from build123d import *

# Parameters (mm, degrees)
F1_DEPTH  = 20
F3_DEPTH  = 4
F5_DEPTH  = 1
F7_DEPTH  = 20.001
F10_W     = 15
F10_H     = 9.1
F11_DEPTH = 1
F8_R      = 3.75
F12_DEPTH = 10


# Not quite as in the source:
# - a pattern or mirror of a feature is missing from the dataset's text; its kind, count and spacing are read off the source's solid


with BuildPart() as f1:
    # F0 (on Front) → F1 (new body)
    with BuildSketch(Plane.XZ):
        Polygon((-16.45, 3), (-19.25, -1.7), (-18.09, -1.7), (-17.0772340426, 0), (0, 0), (0, 3), align=None)
    extrude(amount=F1_DEPTH)

    # F2 (on face) → F3 (cut)
    with BuildSketch(Plane.XZ.offset(20)):
        Polygon((-16.2, 2), (-0.5, 2), (0, 1.8180148829), (0, 3), (-16, 3), (-16.5, 2.1091910703), align=None)
    f3 = extrude(amount=-F3_DEPTH, mode=Mode.SUBTRACT)

    # F3_copies: F3 across plane
    add(f3.mirror(Plane.ZX.offset(-10)), mode=Mode.SUBTRACT)

    # F4 (on face) → F5 (cut)
    with BuildSketch(Plane.XZ.offset(20)):
        Polygon((0, 0), (0, 1.8180148829), (-0.5, 2), (-16.2, 2), (-16.5, 2.1091910703), (-17.683862779, 0), align=None)
    f5 = extrude(amount=-F5_DEPTH, mode=Mode.SUBTRACT)

    # F5_copies: F5 across plane
    add(f5.mirror(Plane.ZX.offset(-10)), mode=Mode.SUBTRACT)

    # F6 (on face) → F7 (cut, through all)
    with BuildSketch(Plane.XZ.offset(20)):
        Polygon((-18.67, -1.7), (-18.09, -1.7), (-17.0772340426, 0), (-17.683862779, 0), align=None)
    extrude(amount=-F7_DEPTH, mode=Mode.SUBTRACT)

    # F10 (on face) → F11 (cut)
    with BuildSketch(Plane(origin=(0, 0, 0), x_dir=(1, 0, 0), z_dir=(0, 0, -1))):
        with Locations((-9, 10)):
            Rectangle(F10_W, F10_H)
    extrude(amount=-F11_DEPTH, mode=Mode.SUBTRACT)

    # F8 (on face) → F12 (join)
    with BuildSketch(Plane.XY.offset(3)):
        with Locations((-8.225, -10)):
            Circle(F8_R)
    extrude(amount=F12_DEPTH)


solid = f1.part
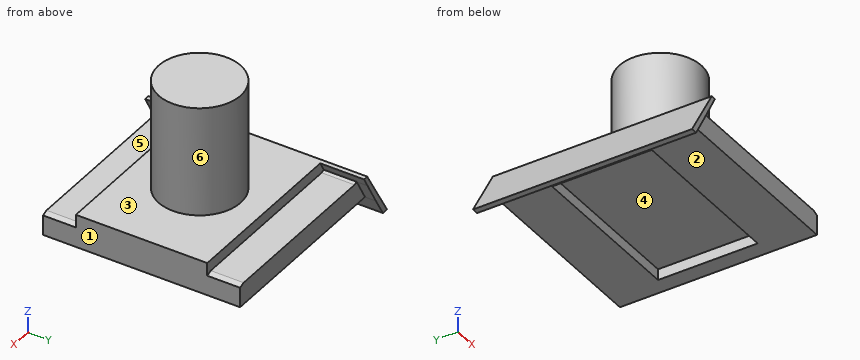
The model under review builds one solid part; all positions refer to its coordinate system, in mm. Face numbers are marked on the shaded views. A direction names the side the tool comes from. Round coordinates to 2 decimals unless told otherwise and drop trailing zeros. Loops run counter-clockwise (first coordinate to the right, second up) from the corner with the lowest first, then second, coordinate; pieces in that order, holes last. Notation, with made-up numbers: (42, 60) -> (94, 60) arc R19 ccw to (94, 94) -> close; hole circle Ø11 at (85, -31.5). An arc over 180 degrees is marked (long way). One line per question, with ' | ' between items. Start each with the question number.
Item 1: Add section B-B, the plane y = -10. Write out the cut boundary in (x, z) (3 decimals).
Item 2: Draft analysis for pull direction Y (two halves, no side actions). For the marked faces 4, 5 and 6, state which applies: +Y half, -Y half, draft (parallel to the pull), parting line (faces both ways), or undercut.
Item 3: Wall thickness on line 1 along Y through (x, z) = (-12.25, 0.25); line 2 along Y through (x, z) = (-3.75, 1.5); line 3 along Z through (x, y) = (-6.75, -18.75): over which ranges is each line inside the solid? List them lowest first. Write a range as [from, to].
Item 4: Machinability: for the marked faces 1, 2 and 3, which of the approach directions +Z, -Z, +X, -X, +Y, -Y give a long, thin tool a straight path to every point of the face, cutting with its end or side? Answer none if there is none.
Item 5: For pin 1 (0.6 mm diameter, centred on x = -13, z = 1, fed in from +Y); pin 2 (2.5 mm diameter, centred on x = -7.5, y = -10, fed in from -Z); pin 3 (4 mm diameter, centred on x = -12, z = 10.5, fed in from -Y), all flat-tipped, find the tip position at first contact; note any pin that passes through.
Item 6: Add section D-D, the plane z = 9.5. Write out the cut boundary in (x, y) (3 decimals), then the cut area to 3 significant figures.
Item 7: Add section A-A, the plane x = -15. Write out the cut boundary in (y, z), then the cut area to 3 significant figures.
Item 8: Add section C-C, the plane z = 0.5. Write out the cut boundary in (x, y).
Return value:
1) outline: (-19.25, -1.7) -> (-18.67, -1.7) -> (-17.684, 0) -> (-16.5, 0) -> (-16.5, 1) -> (-1.5, 1) -> (-1.5, 0) -> (0, 0) -> (0, 3) -> (-4.475, 3) -> (-4.475, 13) -> (-11.975, 13) -> (-11.975, 3) -> (-16.45, 3) -> close
2) face 4: undercut | face 5: draft | face 6: parting line
3) line 1: y = [-19, -14.55], [-5.45, -1] | line 2: y = [-19, -1] | line 3: z = [0, 2]
4) face 1: +Z, -Z, +X, +Y, -Y | face 2: -Z, +X, +Y, -Y | face 3: +Z
5) pin 1: stops at y = -1 | pin 2: stops at z = 1 | pin 3: stops at y = -13.3
6) outline: circle Ø7.5 at (-8.225, -10) | area: 44.2 mm2
7) outline: (-19, 0) -> (-14.55, 0) -> (-14.55, 1) -> (-5.45, 1) -> (-5.45, 0) -> (-1, 0) -> (-1, 2) -> (-4, 2) -> (-4, 3) -> (-16, 3) -> (-16, 2) -> (-19, 2) -> close | area: 38.9 mm2
8) outline: (-17.94, -20) -> (-17.4, -20) -> (-17.4, -19) -> (0, -19) -> (0, -1) -> (-17.4, -1) -> (-17.4, 0) -> (-17.94, 0) -> close; hole (-16.5, -14.55) -> (-1.5, -14.55) -> (-1.5, -5.45) -> (-16.5, -5.45) -> close
